Could you check a few things on this model? Use its own coordinates, in mm. Face numbers are marked on the shaded views. A direction names the side the tool comes from. Give positions to 0.01 mm unless a question says otherwise; leave off trailing zeros. Write each loop counter-clockwise with the first axis right and the second up, starting at its lowest first coordinate (ties: lowest second). Pieces come first, ordered by that corner, then holes. Notation, with made-up numbers: M 5.5,77 L 25.5,77 A26 cw 25.5,98 Z; hole C -1,-4.5 d10. An arc over 180 degrees is marked long. Answer as CSV lines item,"result". Start each with the question number.
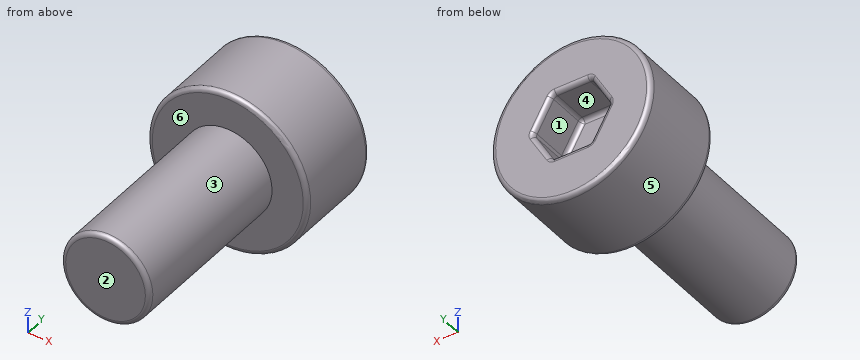
from build123d import *

# Parameters (mm, degrees)
SKETCH1_R           = 2
BOSS_EXTRUDE1_DEPTH = 8
SKETCH2_R           = 3.61
BOSS_EXTRUDE2_DEPTH = 4
CUT_EXTRUDE1_DEPTH  = 2
FILLET1_R           = 0.2


with BuildPart() as part:
    # Sketch1 → Boss-Extrude1 (new body)
    with BuildSketch(Plane(origin=(0, 0, 0), x_dir=(1, 0, 0), z_dir=(0, 1, 0))):
        with Locations(Location((0, 0, 0), (0, 0, 270))):
            Circle(SKETCH1_R)
    extrude(amount=-BOSS_EXTRUDE1_DEPTH)

    # Sketch2 → Boss-Extrude2 (add)
    with BuildSketch(Plane(origin=(0, 0, 0), x_dir=(1, 0, 0), z_dir=(0, 1, 0))):
        with Locations(Location((0, 0, 0), (0, 0, 270))):
            Circle(SKETCH2_R)
    extrude(amount=BOSS_EXTRUDE2_DEPTH)

    # Sketch3 → Cut-Extrude1 (cut)
    with BuildSketch(Plane(origin=(0, 4, 0), x_dir=(1, 0, 0), z_dir=(0, 1, 0))):
        Polygon((1.732050808, 0), (0.866025404, 1.5), (-0.866025404, 1.5), (-1.732050808, 0), (-0.866025404, -1.5), (0.866025404, -1.5), align=None)
    extrude(amount=-CUT_EXTRUDE1_DEPTH, mode=Mode.SUBTRACT)

    # Fillet1
    fillet1_edges = [part.edges().sort_by_distance(p)[0] for p in [
        (1.299038106, 2, 0.75),
        (1.732050808, 3, 0),
        (0, 2, 1.5),
        (0.866025404, 3, 1.5),
        (-1.299038106, 2, 0.75),
        (-0.866025404, 3, 1.5),
        (-1.299038106, 2, -0.75),
        (-1.732050808, 3, 0),
        (0, 2, -1.5),
        (-0.866025404, 3, -1.5),
        (1.299038106, 2, -0.75),
        (0.866025404, 3, -1.5),
        (1.299038106, 4, 0.75),
        (1.299038106, 4, -0.75),
        (0, 4, -1.5),
        (-1.299038106, 4, -0.75),
        (-1.299038106, 4, 0.75),
        (0, 4, 1.5),
        (0, -8, -2),
        (0, 0, -3.61),
        (0, 4, -3.61),
    ]]
    fillet(fillet1_edges, radius=FILLET1_R)


solid = part.part
1. Imagine slicing it at A-A, the plane x = 0. Please give me the cut outline in (y, z), plus the area to 3 significant figures.
2. Thinking about a two-plate mould opening in Z: for the marked faces 4, 5 and 6, which applies, pulls with the +Z half, pulls with the -Z half, needs draft (parallel to the pull), parting line crosses it, or undercut?
3. On a 3-axis mill with a long thin cutter (end or side, diameter ignored), from which of +Z, -Z, +X, -X, +Y, -Y can I reach the whole of each face in a straight line? I mean the marked faces 1, 2 and 3. Say none if no direction works.
4. Please list where these lines run through material, in increasing order: line 1 (Y direction, x = -1.75, z = -2.25); line 2 (Y direction, x = -0.25, z = 0.5); line 3 (Z direction, x = -1.25, y = 3.25).
5. Imagine slicing it at B-B, the plane y = -5. Please give me the cut outline in (x, z), plus the area to 3 significant figures.
6. Will these pins go through, and if not, where does the flat tip stop? P1, Ø1, axis at x = 0, y = -2.5, coming from the -Z side; P2, Ø1.3, axis at x = -0.5, z = -0.5, coming from the +Y side; P3, Ø1, axis at y = -1.5, z = 1.5, coming from the -X side; P4, Ø1, axis at y = -3, z = 3, coming from the -X side.
Solutions:
1,outline,"M -8,-1.8 A0.2 ccw -7.8,-2 L 0,-2 L 0,-3.41 A0.2 ccw 0.2,-3.61 L 3.8,-3.61 A0.2 ccw 4,-3.41 L 4,-1.7 A0.2 ccw 3.8,-1.5 L 2.2,-1.5 A0.2 cw 2,-1.3 L 2,1.3 A0.2 cw 2.2,1.5 L 3.8,1.5 A0.2 ccw 4,1.7 L 4,3.41 A0.2 ccw 3.8,3.61 L 0.2,3.61 A0.2 ccw 0,3.41 L 0,2 L -7.8,2 A0.2 ccw -8,1.8 Z"
1,area,"54.8 mm²"
2,face 4,"undercut"
2,face 5,"parting line crosses it"
2,face 6,"needs draft"
3,face 1,"+Y"
3,face 2,"+Z, -Z, +X, -X, -Y"
3,face 3,"-Y"
4,line 1,"0 to 4"
4,line 2,"-8 to 2"
4,line 3,"-3.39 to -0.83, 0.83 to 3.39"
5,outline,"C 0,0 d4"
5,area,"12.6 mm²"
6,P1,"z = -2"
6,P2,"y = 2"
6,P3,"x = -1.73"
6,P4,"through"
